from build123d import *

# Parameters (mm, degrees)
SKETCH1_W           = 94.24092637
SKETCH1_H           = 65.39427142
BOSS_EXTRUDE1_DEPTH = 5
BOSS_EXTRUDE2_DEPTH = 94.24092637
SKETCH4_R           = 4.5
CUT_EXTRUDE1_DEPTH  = 94.24092637
CUT_EXTRUDE2_START  = -4.69
SKETCH4_4_R         = 6.5
CUT_EXTRUDE2_DEPTH  = 94.24092637
SKETCH3_R           = 3
CUT_EXTRUDE3_DEPTH  = 94.24092637
CUT_EXTRUDE4_START  = -4.5
SKETCH3_3_R         = 4.75
CUT_EXTRUDE4_DEPTH  = 94.24092637


with BuildPart() as part:
    # Sketch1 → Boss-Extrude1 (new body)
    with BuildSketch(Plane.XY):
        with Locations((47.120463185, -32.69713571)):
            Rectangle(SKETCH1_W, SKETCH1_H)
    extrude(amount=BOSS_EXTRUDE1_DEPTH)

    # Sketch2 → Boss-Extrude2 (add)
    with BuildSketch(Plane(origin=(94.24092637, 0, 0), x_dir=(0, 0, -1), z_dir=(1, 0, 0))):
        Polygon((-5, -65.39427142), (-28.80156829, -65.39427142), (-5, 0), align=None)
    extrude(amount=-BOSS_EXTRUDE2_DEPTH)

    # Sketch4 → Cut-Extrude1 (cut)
    with BuildSketch(Plane(origin=(0, 0, 0), x_dir=(-1, 0, 0), z_dir=(0, 0, -1))):
        with Locations((-64.990115154, -26.926235979)):
            Circle(SKETCH4_R)
        with Locations((-28.021847985, -36.1434602)):
            Circle(SKETCH4_R)
    extrude(amount=-CUT_EXTRUDE1_DEPTH, mode=Mode.SUBTRACT)

    # Sketch4_4 → Cut-Extrude2 (cut)
    with BuildSketch(Plane(origin=(0, 0, 0), x_dir=(-1, 0, 0), z_dir=(0, 0, -1)).offset(CUT_EXTRUDE2_START)):
        with Locations((-64.990115154, -26.926235979)):
            Circle(SKETCH4_4_R)
        with Locations((-28.021847985, -36.1434602)):
            Circle(SKETCH4_4_R)
    extrude(amount=-CUT_EXTRUDE2_DEPTH, mode=Mode.SUBTRACT)

    # Sketch3 → Cut-Extrude3 (cut)
    with BuildSketch(Plane(origin=(0, 1.606969024, 4.415111108), x_dir=(1, 0, 0), z_dir=(0, 0.34202014334590697, 0.9396926207785422))):
        with Locations(Location((47.20092637, -35.257197457, 0), (0, 0, 270))):
            Circle(SKETCH3_R)
        with Locations(Location((17.20092637, -50.257197457, 0), (0, 0, 270))):
            Circle(SKETCH3_R)
        with Locations(Location((17.20092637, -20.257197457, 0), (0, 0, 270))):
            Circle(SKETCH3_R)
        with Locations(Location((77.20092637, -20.257197457, 0), (0, 0, 270))):
            Circle(SKETCH3_R)
        with Locations(Location((77.20092637, -50.257197457, 0), (0, 0, 270))):
            Circle(SKETCH3_R)
    extrude(amount=-CUT_EXTRUDE3_DEPTH, mode=Mode.SUBTRACT)

    # Sketch3_3 → Cut-Extrude4 (cut)
    with BuildSketch(Plane(origin=(0, 1.606969024, 4.415111108), x_dir=(1, 0, 0), z_dir=(0, 0.34202014334590697, 0.9396926207785422)).offset(CUT_EXTRUDE4_START)):
        with Locations(Location((17.20092637, -20.257197457, 0), (0, 0, 270))):
            Circle(SKETCH3_3_R)
        with Locations(Location((17.20092637, -50.257197457, 0), (0, 0, 270))):
            Circle(SKETCH3_3_R)
        with Locations(Location((47.20092637, -35.257197457, 0), (0, 0, 270))):
            Circle(SKETCH3_3_R)
        with Locations(Location((77.20092637, -20.257197457, 0), (0, 0, 270))):
            Circle(SKETCH3_3_R)
        with Locations(Location((77.20092637, -50.257197457, 0), (0, 0, 270))):
            Circle(SKETCH3_3_R)
    extrude(amount=-CUT_EXTRUDE4_DEPTH, mode=Mode.SUBTRACT)


solid = part.part
Verification items for the finished model (mm, model axes). A direction names the side the tool comes from. Give positions to 0.01 mm unless a question says otherwise; leave off trailing zeros. Order: outer loops, then holes, each group sorted by start corner. A loop starts at its lowest first (then second) coordinate and runs counter-clockwise, first axis right, second up. Notation, with made-up numbers: M 80.5,-12 L 133.5,-12 A22 cw 133.5,21 Z; hole C 62.5,15.5 d8. An arc over 180 degrees is marked long. Answer as a JSON object with one key per item and string values. Group by question number.
1) Mould release check, pull along Z, two halves, no side actions. Record for faces 1 (the face through (69.4, -25.4, 4.69)), 2 (the face through (29.43, -42.49, 10.76)), 3 (the face through (15.382, -24.306, 5.278)): released by +Z, released by -Z, zero draft, split by the parting line, or undercut.
2) Cross-section at A-A (x = 64). Enter the section's corners in (y, z), then the cut area to 3 significant figures.
3) Cross-section at D-D (x = 36). Enter the section's corners in (y, z).
4) Cross-section at C-C (z = 2). Give the number of separate pieces and of enclosed holes in the cut face, then the cut area to 3 significant figures.
5) Depth check by flat-ended pin: pin 1 Ø8 at (x, y) = (28.02, -36.14) entering from -Z; pin 2 Ø17 at (x, y) = (64.99, -26.93) entering from +Z; pin 3 Ø10.5 at (x, y) = (63, -27.5) entering from +Z; pin 4 Ø3 at (x, y) = (69.5, -29) entering from +Z. Enter the tip coordinate at first touch or a pass-through.
6) Access from +Z, -Z, +X, -X, +Y, -Y to the whole of each face (thin tool, end or side, straight path). Record for faces 4 (the face through (16.212, -50.072, 18.436)), 5 (the face through (61.991, -32.693, 9.476)), 6 (the face through (46, 0, 2)).
7) Scan lines: line 1 along X through (y, z) = (-45, 13.75); line 2 along X through (y, z) = (-47.5, 9.5); line 3 along X through (y, z) = (-29, 13.25). Record each from-to range of solid material in increasing order. Write a range as [from, to].
8) Cross-section at B-B (x = 76). Enter the section's corners in (y, z).
Result sheet:
{
 "1": {"face 1": "released by +Z", "face 2": "zero draft", "face 3": "undercut"},
 "2": {"outline": "M -65.39,0 L -31.32,0 L -31.32,4.69 L -33.35,4.69 L -33.35,17.14 L -65.39,28.8 Z; M -22.54,0 L 0,0 L 0,5 L -20.5,12.46 L -20.5,4.69 L -22.54,4.69 Z", "area": "934 mm2"},
 "3": {"outline": "M -65.39,0 L 0,0 L 0,5 L -65.39,28.8 Z"},
 "4": {"separate pieces": "1", "enclosed holes": "7", "area": "5,660 mm2"},
 "5": {"pin 1": "passes through", "pin 2": "stops at z = 17.9", "pin 3": "stops at z = 16.87", "pin 4": "stops at z = 4.69"},
 "6": {"face 4": "none", "face 5": "+Z", "face 6": "+Z, -Z, +X, -X, +Y"},
 "7": {"line 1": "x = [0, 13.75], [20.65, 73.75], [80.65, 94.24]", "line 2": "x = [0, 13.09], [21.32, 73.09], [81.32, 94.24]", "line 3": "x = [0, 58.83], [71.15, 94.24]"},
 "8": {"outline": "M -65.39,0 L -58.37,0 L -51.48,18.95 L -49.74,18.32 L -48.2,22.54 L -65.39,28.8 Z; M -48.59,0 L -26.45,0 L -23.29,8.69 L -21.55,8.06 L -20.01,12.28 L -43.04,20.66 L -44.58,16.44 L -42.84,15.8 Z; M -16.67,0 L 0,0 L 0,5 L -14.85,10.4 L -16.38,6.17 L -14.65,5.54 Z"}
}
